Here's how the part is built. I have some questions about the finished solid (model axes, mm). Face numbers are marked on the shaded views. A direction names the side the tool comes from. Round coordinates to 2 decimals unless told otherwise and drop trailing zeros. Loops run counter-clockwise (first coordinate to the right, second up) from the corner with the lowest first, then second, coordinate; pieces in that order, holes last. Notation, with made-up numbers: (67.25, -38.5) -> (121.25, -38.5) arc R9 ccw to (121.25, -34.5) -> close; hole circle Ø8 at (-29, 21). An arc over 180 degrees is marked (long way). Use one line per item in the form item = value. Start each with the question number.
Item 1: If we section it at B-B (x = -51): Write out the boundary of the cut face in (y, z).
Item 2: Thinking about a two-plate mould opening in Z: for the marked faces 1, 2 and 3, which applies, released by +Z, released by -Z, zero draft, split by the parting line, or undercut?
Item 3: I'm going to push flat-ended pins straight in: pin 1 Ø5 at (x, z) = (42.5, -65.5) entering from +Y; pin 2 Ø1.5 at (x, z) = (-4, -9.5) entering from +Y; pin 3 Ø21 at (x, z) = (-55.5, -40.5) entering from +Y. Where does each tip first touch, or does it pass through?
Item 4: If we section it at A-A (x = 57.15): Write out the boundary of the cut face in (y, z) (3 decimals).
Item 5: For the marked faces 4 and 5, which set-ups out of +Z, -Z, +X, -X, +Y, -Y let a thin tool reach every point of the face, with its end or its side?
Item 6: If we section it at C-C (z = -45): State how many separate pieces and enclosed holes the cut face has, then the cut area to 3 significant figures.
Item 7: If I drill on L1, parallel to X at y = 62.75, z = -38.1 (3 decimals); L2, parallel to X at y = 65, z = -40; L3, parallel to Z at x = -57, y = 60, over which ranges is the centre line in solid material (lowest first)? Write a range as [from, to].
Item 8: If we section it at D-D (x = -28): Write out the boundary of the cut face in (y, z).
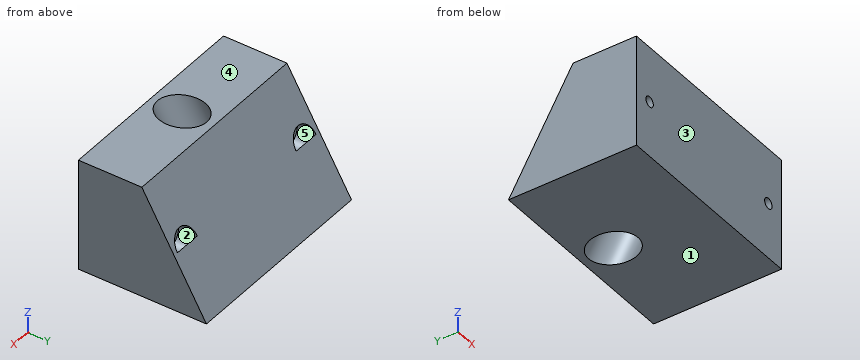
Autodesk Inventor part; units mm, degrees
ref_plane "Work Plane1" through (0, 0, -76.2) normal (0, 0, 1) x (1, 0, 0)
ref_plane "Work Plane2" through (-69.85, 65.177, -38.1) normal (0, -0.5, 0.866) x (1, 0, 0)
ref_plane "YZ Plane" through (0, 0, 0) normal (1, 0, 0) x (0, 1, 0)
sketch "Sketch2" plane through (0, 0, 0) normal (0, 0, 1) x (1, 0, 0)
  line L0 (0, 0) -> (69.85, 0)
  line L1 (69.85, 0) -> (69.85, 43.18)
  line L2 (69.85, 43.18) -> (0, 43.18)
  line L3 (0, 0) -> (0, 43.18) construction
  line L4 (0, 0) -> (-69.85, 0)
  line L5 (-69.85, 0) -> (-69.85, 43.18)
  line L6 (-69.85, 43.18) -> (0, 43.18)
  dimension "d2" = 69.85
  dimension "frontHeight" = 43.18
ref_plane "Work Plane1" through (0, 0, -76.2) normal (0, 0, 1) x (1, 0, 0)
sketch "Sketch3" plane through (0, 0, -76.2) normal (0, 0, 1) x (1, 0, 0)
  line L0 (0, 0) -> (69.85, 0)
  line L1 (69.85, 0) -> (69.85, 87.1741)
  line L2 (69.85, 87.1741) -> (0, 87.1741)
  line L3 (0, 0) -> (0, 87.1741) construction
  line L4 (0, 0) -> (-69.85, 0)
  line L5 (-69.85, 0) -> (-69.85, 87.1741)
  line L6 (-69.85, 87.1741) -> (0, 87.1741)
  dimension "d5" = 69.85
  dimension "rearHeight" = 87.1741
loft "Loft1" add profiles "Sketch2", "Sketch3"
sketch "Sketch4" plane through (69.85, 0, -76.2) normal (1, 0, 0) x (0, 0, -1)
  line L0 (-76.2, 43.18) -> (0, 87.1741) construction
  line L1 (-76.2, 43.18) -> (0, 43.18) construction
  line L2 (0, 0) -> (0, 87.1741) construction
  point P0 (-76.2, 0)
  dimension "d11" = 30
sketch "Sketch5" plane through (-69.85, 43.18, 0) normal (0, 0.866, 0.5) x (1, 0, 0)
  line L0 (0, 0) -> (0, 87.9882) construction
  line L1 (0, 43.9941) -> (139.7, 43.9941) construction
  line L2 (139.7, 0) -> (139.7, 87.9882) construction
  point P0 (69.85, -21.59)
ref_plane "Work Plane2" through (-69.85, 65.177, -38.1) normal (0, -0.5, 0.866) x (1, 0, 0)
sketch "Sketch6" plane through (-69.85, 65.177, -38.1) normal (0, -0.5, 0.866) x (1, 0, 0)
  circle A0 centre (69.85, -19.05) radius 14.605
  line L0 (139.7, 0) -> (0, 0)
  point P0 (69.85, -37.395)
  dimension "holeDiameter" = 29.21
  dimension "centerLineForHole" = 19.05
extrude "Extrusion1" cut sketch "Sketch6" along normal through all both and the other way through all
ref_plane "centerLineForHoleWork Plane" through (-69.85, 26.6822, -9.525) normal (0, 0.866, 0.5) x (1, 0, 0)
ref_plane "screwHoleWork Plane" through (69.85, 65.177, -38.1) normal (0, 1, 0) x (-1, 0, 0)
sketch "Sketch7" plane through (69.85, 65.177, -38.1) normal (0, 1, 0) x (-1, 0, 0)
  line L0 (0, -38.1) -> (139.7, -38.1) construction
  line L1 (69.85, -38.1) -> (69.85, 38.1) construction
  point P0 (127, 0)
  point P1 (12.7, 0)
  dimension "d18" = 57.15
  dimension "d19" = 57.15
hole "Hole1" at (-57.15, 65.177, -38.1) at (57.15, 65.177, -38.1) direction (0, -1, 0) diameter 7.1374 end through all counterbore diameter 19.05 counterbore depth 12.7
equation "\"d2\" = 0.5 * width"
equation "\"d5\" = 0.5 * width"
equation "\"rearHeight\" = frontHeight + 0.57735 * depth"
equation "\"width\" = 139.7"
equation "\"d4\" = -depth"
equation "\"depth\" = 76.2"
equation "\"d17\" = -centerLineForHole"
properties part number "swallowMountV02"
Values found:
q1.outline = (0, -76.2) -> (87.17, -76.2) -> (65.18, -38.1) -> (65.18, -45.37) -> (52.48, -45.37) -> (52.48, -30.83) -> (60.98, -30.83) -> (43.18, 0) -> (0, 0) -> close
q2.face_1 = released by -Z
q2.face_2 = undercut
q2.face_3 = zero draft
q3.pin_1 = 82.44
q3.pin_2 = 49.1
q3.pin_3 = 72.62
q4.outline = (0, -76.2) -> (87.174, -76.2) -> (65.177, -38.1) -> (65.177, -47.625) -> (52.477, -47.625) -> (52.477, -41.669) -> (0, -41.669) -> close; (0, -34.531) -> (52.477, -34.531) -> (52.477, -28.575) -> (59.678, -28.575) -> (43.18, 0) -> (0, 0) -> close
q5.face_4 = +Z, +X, -X, +Y, -Y
q5.face_5 = none
q6.separate_pieces = 1
q6.enclosed_holes = 3
q6.area = 8,550 mm2
q7.L1 = [-69.85, -66.675], [-47.625, 47.625], [66.675, 69.85]
q7.L2 = [-69.85, -66.48], [-47.82, 47.82], [66.48, 69.85]
q7.L3 = [-76.2, -47.62]
q8.outline = (0, -76.2) -> (87.17, -76.2) -> (43.18, 0) -> (0, 0) -> close
